Could you check a few things on this drawing? It's one solid part, dimensions in mm from its lowest x, y, z. A direction names the side the tool comes from. Give positions to 0.01 mm unless a question says otherwise; leave off trailing zeros. Order: outer loops, then holes, each group sorted by start corner. A loop starts at its lowest first (then second) coordinate and runs counter-clockwise, first axis right, second up. Notation, with made-up numbers: M -10.5,-18 L 20.5,-18 A19 cw 20.5,9 Z; hole C -37,32.5 d11. An arc over 180 degrees is marked long. One line per item, written item: value. Start each with the question number.
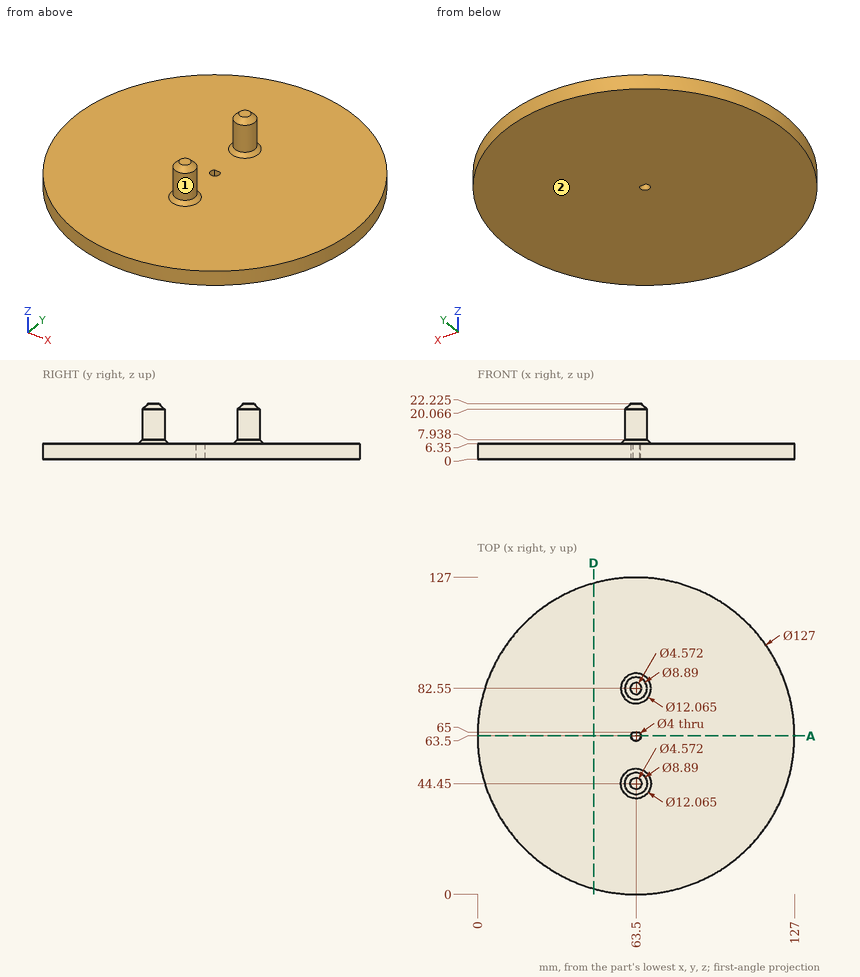
Item 1: Will these pins go through, and if not, where does the flat tip stop? P1, Ø10, axis at x = 95.5, z = 4, coming from the +Y side (1 decimal); P2, Ø4, axis at y = 25, z = 5, coming from the -X side; P3, Ø5, axis at x = 102.5, y = 94.5, coming from the +Z side.
Item 2: For the marked faces 1 and 2, which set-ups out of +Z, -Z, +X, -X, +Y, -Y let a thin tool reach every point of the face, with its end or its side?
Item 3: Please list where these lines run through material, in increasing order: probe 1 along Y at (x, z) = (63.5, 1.5); probe 2 along Z at (x, y) = (27, 44.5); probe 3 along Y at (x, z) = (61.5, 9). Write a range as [from, to].
Item 4: I want a section at A-A on y = 63.5. Write out the boundary of the cut face in (x, z).
Item 5: I want a section at D-D on x = 46.5. Write out the boundary of the cut face in (y, z).
Answer below:
1. P1: stops at y = 121
1. P2: stops at x = 11.54
1. P3: stops at z = 6.35
2. face 1: +Z
2. face 2: -Z, +X, -X, +Y, -Y
3. probe 1: y = [0, 61.5], [65, 127]
3. probe 2: z = [0, 6.35]
3. probe 3: y = [40.48, 48.42], [78.58, 86.52]
4. outline: M 0,0 L 61.5,0 L 61.5,6.35 L 0,6.35 Z; M 65.5,0 L 127,0 L 127,6.35 L 65.5,6.35 Z
5. outline: M 2.32,0 L 124.68,0 L 124.68,6.35 L 2.32,6.35 Z
